Verification items for this drawing (mm, ordinates from the low corner). A direction names the side the tool comes from. Give positions to 0.01 mm unless a question says otherwise; leave off trailing zeros. Loops run counter-clockwise (first coordinate to the right, second up) from the corner with the lowest first, then second, coordinate; pieces in that order, holes last. Notation, with made-up numbers: (64, 47) -> (88, 47) arc R35 ccw to (88, 85) -> close; hole circle Ø1 at (78.25, 25). An arc over 180 degrees is marked (long way). Use one line per item in the form item = value. Start each with the question number.
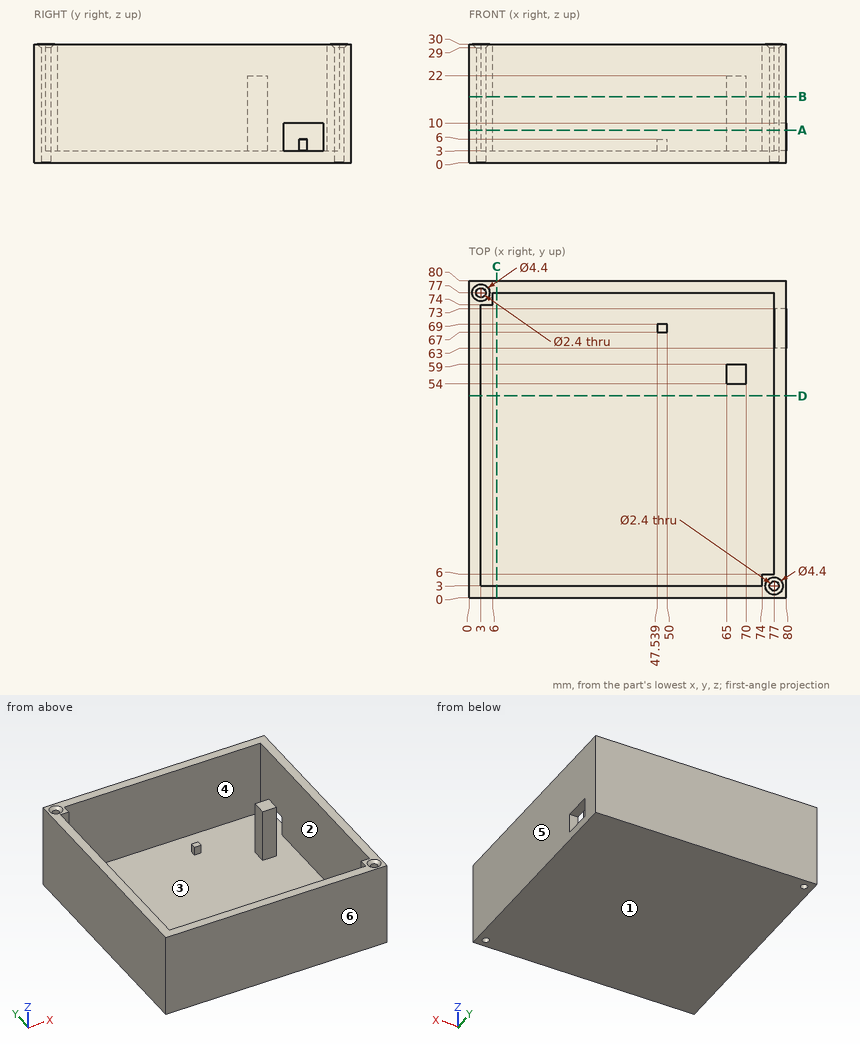
Item 1: Sectioned sample at B-B, the plane z = 16.75. Enter the section's corners in (x, y), and give its area (3 significant figures).
Item 2: Material ranges on line 1 (X direction, y = 45.5, z = 13.75); line 2 (Z direction, x = 71, y = 42), recorded low to high.
Item 3: Sectioned sample at C-C, the plane x = 7. Enter the section's corners in (y, z), and give its area (3 significant figures).
Item 4: Tool access check on the marked faces 1 and 2. Record the directions out of +Z, -Z, +X, -X, +Y, -Y that give a thin tool (end or side, any length) a straight path to the whole face; none if there is none.
Item 5: Sectioned sample at A-A, the plane z = 8.25. Enter the section's corners in (x, y).
Item 6: Draft check along X on the marked faces 3, 4, 5 and 6. Enter one of: +X half, -X half, draft (parallel to the pull), parting line (faces both ways), or undercut.
Item 7: Gauge pin test, flat ends, axial feed: pin 1 Ø4 at (x, y) = (3, 77) entering from +Z; pin 2 Ø2 at (x, y) = (48.5, 68.5) entering from +Z; pin 3 Ø2 at (x, y) = (31, 52) entering from +Z. Record the tip position at first contact, or that the pin passes through.
Outcome:
q1.outline = (0, 0) -> (80, 0) -> (80, 80) -> (0, 80) -> close; (65, 54) -> (70, 54) -> (70, 59) -> (65, 59) -> close; hole circle Ø2.4 at (3, 77); hole (3, 3) -> (74, 3) -> (74, 6) -> (77, 6) -> (77, 77) -> (6, 77) -> (6, 74) -> (3, 74) -> close; hole circle Ø2.4 at (77, 3)
q1.area = 958 mm^2
q2.line_1 = 0 to 3, 77 to 80
q2.line_2 = 0 to 3
q3.outline = (0, 0) -> (80, 0) -> (80, 30) -> (77, 30) -> (77, 3) -> (3, 3) -> (3, 30) -> (0, 30) -> close
q3.area = 402 mm^2
q4.face_1 = -Z, +X, -X, +Y, -Y
q4.face_2 = +Z
q5.outline = (0, 0) -> (80, 0) -> (80, 63) -> (77, 63) -> (77, 6) -> (74, 6) -> (74, 3) -> (3, 3) -> (3, 74) -> (6, 74) -> (6, 77) -> (77, 77) -> (77, 73) -> (80, 73) -> (80, 80) -> (0, 80) -> close; (65, 54) -> (70, 54) -> (70, 59) -> (65, 59) -> close; hole circle Ø2.4 at (3, 77); hole circle Ø2.4 at (77, 3)
q6.face_3 = undercut
q6.face_4 = undercut
q6.face_5 = +X half
q6.face_6 = draft
q7.pin_1 = 29.8
q7.pin_2 = 6
q7.pin_3 = 3
